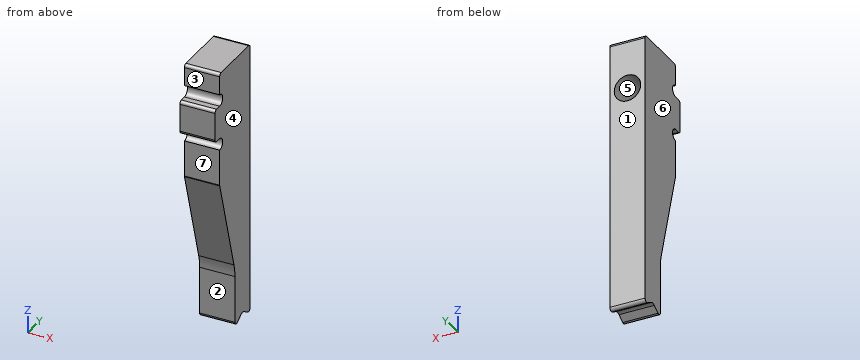
from build123d import *

# Parameters (mm, degrees)
ESQUISSE1_W             = 6
ESQUISSE1_H             = 5
BOSS_EXTRU_1_DEPTH      = 8.5
ESQUISSE5_W             = 6
ESQUISSE5_H             = 5
BOSS_EXTRU_3_DEPTH      = 30
ENL_V_MAT_EXTRU_2_DEPTH = 40.044846011
ESQUISSE7_W             = 6
ESQUISSE7_H             = 17
BOSS_EXTRU_4_DEPTH      = 5
ESQUISSE2_R             = 2.25
ENL_V_MAT_EXTRU_1_DEPTH = 40.890475054
ESQUISSE9_W             = 6
ESQUISSE9_H             = 5.7
BOSS_EXTRU_6_DEPTH      = 1.5
ENL_V_MAT_EXTRU_3_DEPTH = 40.990623901
CHANFREIN2_SIZE         = 20
CHANFREIN2_SIZE_2       = 5.734907715
CONG_1_R                = 0.5
CONG_2_R                = 1
CONG_3_R                = 8


with BuildPart() as part:
    # Esquisse1 → Boss.-Extru.1 (new, symmetric)
    with BuildSketch(Plane.XY):
        Rectangle(ESQUISSE1_W, ESQUISSE1_H)
    extrude(amount=BOSS_EXTRU_1_DEPTH, both=True)

    # Esquisse5 → Boss.-Extru.3 (add)
    with BuildSketch(Plane(origin=(-2.5, 0, -8.5), x_dir=(1, 0, 0), z_dir=(0, 0, 1))):
        with Locations((2.5, 0)):
            Rectangle(ESQUISSE5_W, ESQUISSE5_H)
    extrude(amount=-BOSS_EXTRU_3_DEPTH)

    # Esquisse6 → Enlèv. mat.-Extru.2 (cut, through all)
    with BuildSketch(Plane(origin=(3, 0, 0), x_dir=(0, 0, -1), z_dir=(1, 0, 0))):
        Polygon((38.5, 2.5), (37.056624327, 0), (38.5, -2.5), align=None)
    extrude(amount=-ENL_V_MAT_EXTRU_2_DEPTH, mode=Mode.SUBTRACT)

    # Esquisse7 → Boss.-Extru.4 (add)
    with BuildSketch(Plane.XZ.offset(2.5)):
        Rectangle(ESQUISSE7_W, ESQUISSE7_H)
    extrude(amount=BOSS_EXTRU_4_DEPTH)

    # Esquisse2 → Enlèv. mat.-Extru.1 (cut, through all)
    with BuildSketch(Plane(origin=(0, 2.5, 0), x_dir=(1, 0, 0), z_dir=(0, 1, 0))):
        with Locations(Location((0, 0, 0), (0, 0, 270))):
            Circle(ESQUISSE2_R)
    extrude(amount=-ENL_V_MAT_EXTRU_1_DEPTH, mode=Mode.SUBTRACT)

    # Esquisse9 → Boss.-Extru.6 (add)
    with BuildSketch(Plane.XZ.offset(7.5)):
        Rectangle(ESQUISSE9_W, ESQUISSE9_H)
    extrude(amount=BOSS_EXTRU_6_DEPTH)

    # Esquisse10 → Enlèv. mat.-Extru.3 (cut, through all)
    with BuildSketch(Plane(origin=(3, 0, 0), x_dir=(0, 0, -1), z_dir=(1, 0, 0))):
        with BuildLine():
            Line((-4.85, -7.5), (-2.85, -7.5))
            ThreePointArc((-2.85, -7.5), (-3.85, -6.5), (-4.85, -7.5))
        make_face()
        with BuildLine():
            Line((4.85, -7.5), (2.85, -7.5))
            ThreePointArc((2.85, -7.5), (3.85, -6.5), (4.85, -7.5))
        make_face()
    extrude(amount=-ENL_V_MAT_EXTRU_3_DEPTH, mode=Mode.SUBTRACT)

    # Chanfrein2
    # the kernel refuses this chamfer: 20, 5.734907715 mm, written as the material it adds along each edge
    with BuildSketch(Plane(origin=(3, -2.5, -8.5), x_dir=(0, 0.010616657410321303, -0.9999436417045873), z_dir=(-1, 0, 0))) as chanfrein2_piece_1_section:
        Polygon((CHANFREIN2_SIZE * 0.999943641705, CHANFREIN2_SIZE * 0.0106166574103), (-CHANFREIN2_SIZE_2 * 0.0106166574106, CHANFREIN2_SIZE_2 * 0.999943641735), (0, 0), align=None)
    chanfrein2_piece_1 = extrude(amount=6, mode=Mode.PRIVATE)
    chanfrein2_piece_1 = split(chanfrein2_piece_1, bisect_by=Plane(origin=(0, -7.5, -15.61390523), z_dir=(0, 1, 0)), keep=Keep.TOP, mode=Mode.PRIVATE)
    add(chanfrein2_piece_1)

    # Congé1
    cong_1_edges = [part.edges().sort_by_distance(p)[0] for p in [
        (0, -2.5, -38.5),
        (0, 2.5, -38.5),
        (0, -7.5, 8.5),
        (0, -9, 2.85),
        (0, -9, -2.85),
        (0, 2.5, 8.5),
        (0, -7.5, -11.062927781),
    ]]
    fillet(cong_1_edges, radius=CONG_1_R)

    # Congé2
    cong_2_edges = [part.edges().sort_by_distance(p)[0] for p in [
        (0, 0, -37.056624327),
    ]]
    fillet(cong_2_edges, radius=CONG_2_R)

    # Congé3
    cong_3_edges = [part.edges().sort_by_distance(p)[0] for p in [
        (0, -2.5, -28.5),
    ]]
    fillet(cong_3_edges, radius=CONG_3_R)


solid = part.part
Here's how the part is built. I have some questions about the finished solid (model axes, mm). Face numbers are marked on the shaded views. A direction names the side the tool comes from. Round coordinates to 2 decimals unless told otherwise and drop trailing zeros. Loops run counter-clockwise (first coordinate to the right, second up) from the corner with the lowest first, then second, coordinate; pieces in that order, holes last.
1. If we section it at D-D on y = -3.75: Write out the boundary of the cut face in (x, z).
Answer list:
outline: (-3, -24.14) - (3, -24.14) - (3, 8.5) - (-3, 8.5) - close; hole circle Ø4.5 at (0, 0)
2. For P1, Ø3, axis at x = 0.5, z = -8, coming from the -Y side; P2, Ø0.8, axis at x = 0.5, y = -8, coming from the +Z side, each with a flat end and sliding along its axis, tell me the tip position at first contact or that it passes through.
Answer list:
P1: stops at y = -7.5
P2: stops at z = 2.85
3. Which directions (+Z, -Z, +X, -X, +Y, -Y) give clear straight access to the entire face, cutting with the end or side of a thin tool? Please do the marked faces 1, 2 and 3.
Answer list:
face 1: +Z, -Z, +X, -X, +Y
face 2: -Z, +X, -X, -Y
face 3: +Z, +X, -X, -Y
4. If we section it at A-A on z = 0: Write out the boundary of the cut face in (x, y).
Answer list:
outline: (-3, -9) - (3, -9) - (3, 2.5) - (2.25, 2.5) - (2.25, -7.5) - (-2.25, -7.5) - (-2.25, 2.5) - (-3, 2.5) - close
5. If I drill on line 1 along X through (y, z) = (-3.75, 0); line 2 along Z through (x, y) = (1.25, -8.25); line 3 along Y through (x, z) = (-1, -6.5), over which ranges is the centre line in solid material (lowest first)?
Answer list:
line 1: x = -3 to -2.25, 2.25 to 3
line 2: z = -2.85 to 2.85
line 3: y = -7.5 to 2.5
6. If we section it at C-C on y = -8: Write out the boundary of the cut face in (x, z), plus the area to 3 significant figures.
Answer list:
outline: (-3, -2.85) - (3, -2.85) - (3, 2.85) - (-3, 2.85) - close
area: 34.2 mm2
7. If we section it at B-B on x = 0: Write out the boundary of the cut face in (y, z).
Answer list:
outline: (-9, -2.35) arc R0.5 ccw to (-8.5, -2.85) - (-7.5, -2.85) arc R1 cw to (-7.5, -4.85) - (-7.5, -10.99) arc R0.5 ccw to (-7.48, -11.13) - (-2.81, -27.42) arc R8 cw to (-2.5, -29.62) - (-2.5, -37.63) arc R0.5 ccw to (-1.75, -38.07) - (-0.5, -37.35) arc R1 cw to (0.5, -37.35) - (1.75, -38.07) arc R0.5 ccw to (2.5, -37.63) - (2.5, -2.25) - (-7.5, -2.25) - (-7.5, 2.25) - (2.5, 2.25) - (2.5, 8) arc R0.5 ccw to (2, 8.5) - (-7, 8.5) arc R0.5 ccw to (-7.5, 8) - (-7.5, 4.85) arc R1 cw to (-7.5, 2.85) - (-8.5, 2.85) arc R0.5 ccw to (-9, 2.35) - close
8. We'd pull the mould along X, two halves only. Please class the marked faces 4, 5, 6 and 7: +X half, -X half, draft (parallel to the pull), parting line (faces both ways), or undercut.
Answer list:
face 4: +X half
face 5: undercut
face 6: -X half
face 7: draft
